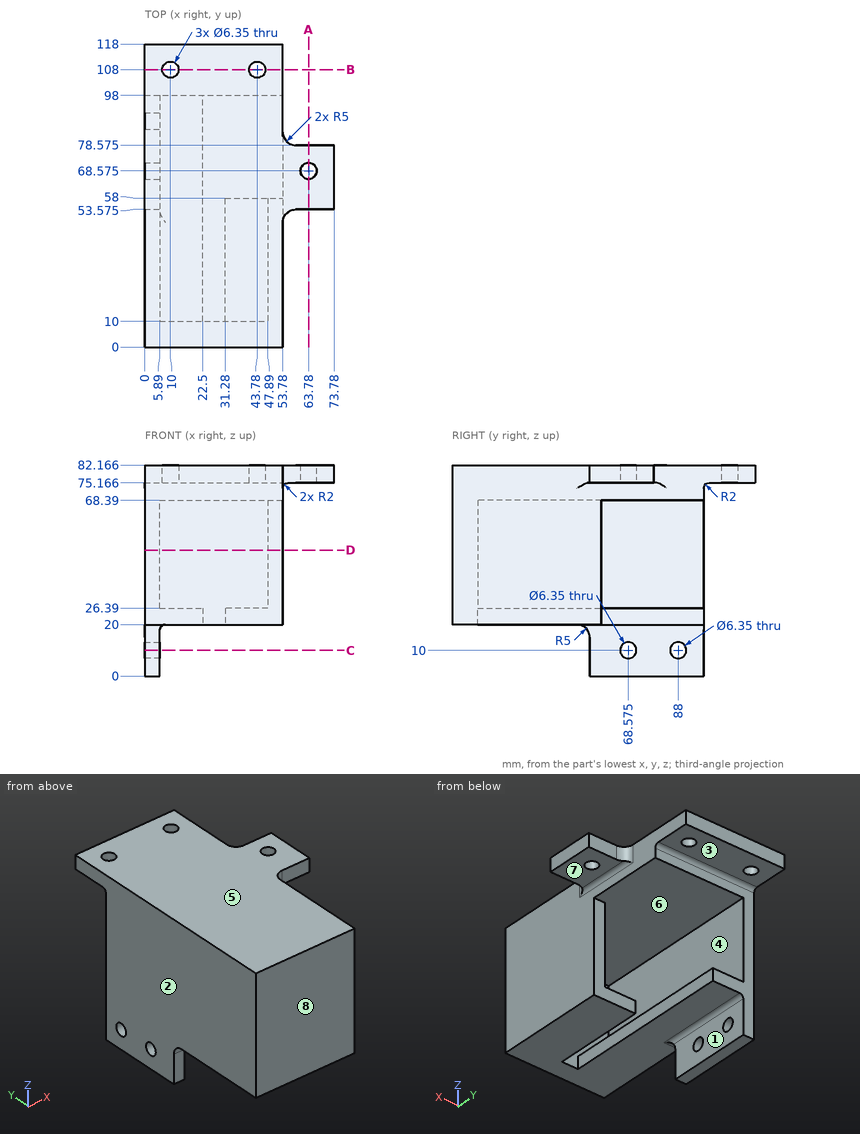
Verification items for this drawing (mm, ordinates from the low corner). A direction names the side the tool comes from. Coordinates: 2 decimals unless noted, no trailing zeros. Order: outer loops, then holes, each group sorted by start corner. A loop starts at its lowest first (then second) coordinate and runs counter-clockwise, first axis right, second up. Notation, with made-up numbers: (26, 33) - (41, 33) arc R16 cw to (41, 45) - close; hole circle Ø6 at (83, -5.5). An arc over 180 degrees is marked (long way). Answer as a JSON object with one key per item and string values. Group by question number.
Item 1: Sectioned sample at D-D, the plane z = 49. Record the cut outline in (x, y), and give its area (3 significant figures).
Item 2: Sectioned sample at C-C, the plane z = 10. Record the cut outline in (x, y) (3 decimals).
Item 3: Depth check by flat-ended pin: pin 1 Ø10 at (x, z) = (9.5, 63) entering from +Y; pin 2 Ø1.5 at (x, y) = (41, 63) entering from -Z; pin 3 Ø1.5 at (y, z) = (65.5, 55) entering from +X. Enter the tip coordinate at first touch or a pass-through.
Item 4: Scan lines: probe 1 along Z at (x, y) = (20, 10.5); probe 2 along Y at (x, z) = (3.6, 10) (3 decimals); probe 3 along X at (y, z) = (56.5, 46). Record each from-to range of solid material in increasing order.
Item 5: Draft check along Z on the marked faces 6, 7 and 8. Enter one of: +Z half, -Z half, draft (parallel to the pull), parting line (faces both ways), or undercut.
Item 6: Sectioned sample at B-B, the plane y = 108. Record the cut outline in (x, z) (3 decimals).
Item 7: Sectioned sample at A-A, the plane x = 63.78. Record the cut outline in (y, z) (3 decimals).
Item 8: Tool access check on the marked faces 1, 2, 3, 4 and 5. Record the directions out of +Z, -Z, +X, -X, +Y, -Y that give a thin tool (end or side, any length) a straight path to the whole face; none if there is none.
Resolved:
{
 "1": {"outline": "(0, 0) - (53.78, 0) - (53.78, 58) - (47.89, 58) - (47.89, 10) - (5.89, 10) - (5.89, 98) - (0, 98) - close", "area": "1,340 mm^2"},
 "2": {"outline": "(0, 53.575) - (5.89, 53.575) - (5.89, 65.4) - (0, 65.4) - close; (0, 71.75) - (5.89, 71.75) - (5.89, 84.825) - (0, 84.825) - close; (0, 91.175) - (5.89, 91.175) - (5.89, 98) - (0, 98) - close"},
 "3": {"pin 1": "y = 98", "pin 2": "z = 68.39", "pin 3": "x = 5.89"},
 "4": {"probe 1": "20 to 26.39, 68.39 to 82.17", "probe 2": "53.575 to 65.4, 71.75 to 84.825, 91.175 to 98", "probe 3": "0 to 5.89, 47.89 to 53.78"},
 "5": {"face 6": "undercut", "face 7": "-Z half", "face 8": "draft"},
 "6": {"outline": "(0, 75.166) - (6.825, 75.166) - (6.825, 82.166) - (0, 82.166) - close; (13.175, 75.166) - (40.605, 75.166) - (40.605, 82.166) - (13.175, 82.166) - close; (46.955, 75.166) - (53.78, 75.166) - (53.78, 82.166) - (46.955, 82.166) - close"},
 "7": {"outline": "(53.575, 75.166) - (65.4, 75.166) - (65.4, 82.166) - (53.575, 82.166) - close; (71.75, 75.166) - (78.575, 75.166) - (78.575, 82.166) - (71.75, 82.166) - close"},
 "8": {"face 1": "-Z, +X, +Y, -Y", "face 2": "+Z, -Z, -X, +Y, -Y", "face 3": "-Z, +X, -X, +Y", "face 4": "+Y", "face 5": "+Z, +X, -X, +Y, -Y"}
}
